Check sheet for the modelled part. Datum: model origin and axes. Units: mm. A direction names the side the tool comes from. Give positions to 0.01 mm unless a question says otherwise; leave off trailing zeros. Loops run counter-clockwise (first coordinate to the right, second up) from the corner with the lowest first, then second, coordinate; pieces in that order, holes last.
```python
from build123d import *

# Parameters (mm, degrees)
PAD_DEPTH          = 6
POCKET_DEPTH       = 3
SKETCH002_W        = 18.4
SKETCH002_H        = 20.85
POCKET001_DEPTH    = 3
SKETCH003_W        = 8.55
SKETCH003_H        = 1.65
POCKET002_DEPTH    = 3
PAD001_DEPTH       = 3
SKETCH005_W        = 127
SKETCH005_H        = 6
PAD002_DEPTH       = 3
SKETCH006_R        = 0.825
POCKET003_DEPTH    = 442.080062
POLARPATTERN_COUNT = 2


with BuildPart() as part:
    # Sketch → Pad (new body)
    with BuildSketch(Plane.XY):
        with BuildLine():
            ThreePointArc((-75, 28.5), (-103.5, 0), (-75, -28.5))
            Line((-75, -28.5), (75, -28.5))
            ThreePointArc((75, -28.5), (103.5, 0), (75, 28.5))
            Line((-75, 28.5), (75, 28.5))
        make_face()
    extrude(amount=PAD_DEPTH)

    # Sketch001 (on Face6 of Pad) → Pocket (cut)
    with BuildSketch(Plane.XY.offset(6)):
        with BuildLine():
            ThreePointArc((-62.5, 6), (-68.5, 0), (-62.5, -6))
            Line((-62.5, -6), (62.5, -6))
            ThreePointArc((62.5, -6), (68.5, 0), (62.5, 6))
            Line((-62.5, 6), (62.5, 6))
        make_face()
    extrude(amount=-POCKET_DEPTH, mode=Mode.SUBTRACT)

    # Sketch002 (on Face5 of Pocket) → Pocket001 (cut)
    with BuildSketch(Plane.XY.offset(6)):
        with Locations((0, -16.425)):
            Rectangle(SKETCH002_W, SKETCH002_H)
    extrude(amount=-POCKET001_DEPTH, mode=Mode.SUBTRACT)

    # Sketch003 (on Face5 of Pocket001) → Pocket002 (cut)
    with BuildSketch(Plane.XY.offset(6)):
        with Locations((0, -27.675)):
            Rectangle(SKETCH003_W, SKETCH003_H)
    extrude(amount=-POCKET002_DEPTH, mode=Mode.SUBTRACT)

    # Sketch004 (on Face5 of Pocket002) → Pad001 (join)
    with BuildSketch(Plane.XY.offset(6)):
        with BuildLine():
            ThreePointArc((-75, 28.5), (-103.5, 0), (-75, -28.5))
            Line((-75, -28.5), (75, -28.5))
            ThreePointArc((75, -28.5), (103.5, 0), (75, 28.5))
            Line((-75, 28.5), (75, 28.5))
        make_face()
        with BuildLine():
            ThreePointArc((-62.5, 6), (-68.5, 0), (-62.5, -6))
            Line((-62.5, -6), (62.5, -6))
            ThreePointArc((62.5, -6), (68.5, 0), (62.5, 6))
            Line((-62.5, 6), (62.5, 6))
        make_face(mode=Mode.SUBTRACT)
    extrude(amount=PAD001_DEPTH)

    # Sketch005 (on Face12 of Pad001) → Pad002 (join)
    with BuildSketch(Plane.XY.offset(9)):
        with BuildLine():
            ThreePointArc((-75, 28.5), (-103.5, 0), (-75, -28.5))
            Line((-75, -28.5), (75, -28.5))
            ThreePointArc((75, -28.5), (103.5, 0), (75, 28.5))
            Line((-75, 28.5), (75, 28.5))
        make_face()
        Rectangle(SKETCH005_W, SKETCH005_H, mode=Mode.SUBTRACT)
    extrude(amount=PAD002_DEPTH)

    # Sketch006 (on Face20 of Pad002) → Pocket003 (cut, through all)
    with BuildSketch(Plane.XY.offset(12)):
        with Locations((-66.64, -7.79)):
            Circle(SKETCH006_R)
        with Locations((-50, -7.79)):
            Circle(SKETCH006_R)
    pocket003 = extrude(amount=-POCKET003_DEPTH, mode=Mode.SUBTRACT)

    # Mirrored: Pocket003 across Sketch006 H_Axis
    add(pocket003.mirror(Plane(origin=(0, 0, 12), x_dir=(0, 0, 1), z_dir=(0, 1, 0))), mode=Mode.SUBTRACT)

    # Mirrored001: Pocket003 across Sketch006 V_Axis
    add(pocket003.mirror(Plane(origin=(0, 0, 12), x_dir=(0, 0, 1), z_dir=(1, 0, 0))), mode=Mode.SUBTRACT)

    # PolarPattern: Pocket003 ×2 about axis
    polarpattern_axis = Axis((0, 0, 12), (0, 0, 1))
    for i in range(1, POLARPATTERN_COUNT):
        add(pocket003.rotate(polarpattern_axis, i * 360 / POLARPATTERN_COUNT), mode=Mode.SUBTRACT)


solid = part.part
```
(1) Material ranges on line 1 (Y direction, x = 50, z = 5.5) (3 decimals); line 2 (Y direction, x = -45.5, z = 11); line 3 (X direction, y = 7.79, z = 4.75) (3 decimals), recorded low to high.
(2) Gauge pin test, flat ends, axial feed: pin 1 Ø6 at (y, z) = (12, 9.5) entering from -X; pin 2 Ø5 at (y, z) = (14.5, 9.5) entering from -X; pin 3 Ø2.5 at (y, z) = (-14.5, 4) entering from +X; pin 4 Ø1.3 at (x, y) = (-50, -7.79) entering from -Z. Record the tip position at first contact, or that the pin passes through.
(3) Section check C-C on y = 22.5. Record the boundary of the cut face in (x, z).
(4) Release check for a two-part mould opening along Z. For faces 1 (the face through (-68.5, 0.1, 6)), 2 (the face through (-1, 0, 0)), 3 (the face through (-103.493, 0.627, 5.916)) record: pulls with the +Z half, pulls with the -Z half, needs draft (parallel to the pull), parting line crosses it, or undercut.
(5) Section check B-B on y = -17.5. Record the boundary of the cut face in (x, z), plus the area to 3 significant figures.
(6) Section check D-D on x = 87. Record the boundary of the cut face in (y, z), plus the area to 3 significant figures.
(7) Section check A-A on x = -47. Record the boundary of the cut face in (y, z).
(8) Access from +Z, -Z, +X, -X, +Y, -Y to the whole of each face (thin tool, end or side, straight path). Record for faces 4 (the face through (68.5, -0.1, 6)), 5 (the face through (-1, -28.5, 7)).
Computed values:
1. line 1: y = -28.5 to -8.615, -6.965 to -6, 6 to 6.965, 8.615 to 28.5
1. line 2: y = -28.5 to -3, 3 to 28.5
1. line 3: x = -102.415 to -67.465, -65.815 to -50.825, -49.175 to 49.175, 50.825 to 65.815, 67.465 to 102.415
2. pin 1: stops at x = -102.04
2. pin 2: stops at x = -100.85
2. pin 3: stops at x = 100.23
2. pin 4: passes through
3. outline: (-92.49, 0) - (92.49, 0) - (92.49, 12) - (-92.49, 12) - close
4. face 1: undercut
4. face 2: pulls with the -Z half
4. face 3: needs draft
5. outline: (-97.49, 0) - (97.49, 0) - (97.49, 12) - (-97.49, 12) - close; hole (-9.2, 3) - (9.2, 3) - (9.2, 6) - (-9.2, 6) - close
5. area: 2,280 mm2
6. outline: (-25.85, 0) - (25.85, 0) - (25.85, 12) - (-25.85, 12) - close
6. area: 620 mm2
7. outline: (-28.5, 0) - (28.5, 0) - (28.5, 12) - (3, 12) - (3, 9) - (6, 9) - (6, 3) - (-6, 3) - (-6, 9) - (-3, 9) - (-3, 12) - (-28.5, 12) - close
8. face 4: none
8. face 5: +Z, -Z, +X, -X, -Y
